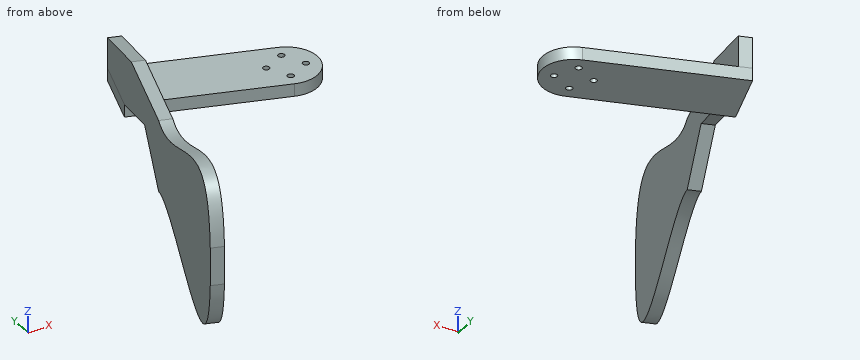
from build123d import *

# Parameters (mm, degrees)
SKETCH2_R           = 10
SKETCH2_R_2         = 1.275
BOSS_EXTRUDE1_DEPTH = 3
SKETCH3_R           = 1.275
BOSS_EXTRUDE2_DEPTH = 5
BOSS_EXTRUDE3_DEPTH = 5


with BuildPart() as part:
    # Sketch2 → Boss-Extrude1 (new body)
    with BuildSketch(Plane.XY):
        Circle(SKETCH2_R)
        with Locations((6.633008125, -2.236784122)):
            Circle(SKETCH2_R_2, mode=Mode.SUBTRACT)
        with Locations((-2.236784122, -6.633008125)):
            Circle(SKETCH2_R_2, mode=Mode.SUBTRACT)
        with Locations((-6.633008125, 2.236784122)):
            Circle(SKETCH2_R_2, mode=Mode.SUBTRACT)
        with Locations((2.236784122, 6.633008125)):
            Circle(SKETCH2_R_2, mode=Mode.SUBTRACT)
    extrude(amount=BOSS_EXTRUDE1_DEPTH)

    # Sketch3 → Boss-Extrude2 (add)
    with BuildSketch(Plane.XY.offset(3)):
        with BuildLine():
            Line((-3.994257361, -11.844657367), (-60.848612721, 7.327777966))
            Line((-60.848612721, 7.327777966), (-52.860097999, 31.0170927))
            Line((-52.860097999, 31.0170927), (3.994257361, 11.844657367))
            ThreePointArc((3.994257361, 11.844657367), (11.844657367, -3.994257361), (-3.994257361, -11.844657367))
        make_face()
        with Locations((6.633008125, -2.236784122)):
            Circle(SKETCH3_R, mode=Mode.SUBTRACT)
        with Locations((-2.236784122, -6.633008125)):
            Circle(SKETCH3_R, mode=Mode.SUBTRACT)
        with Locations((-6.633008125, 2.236784122)):
            Circle(SKETCH3_R, mode=Mode.SUBTRACT)
        with Locations((2.236784122, 6.633008125)):
            Circle(SKETCH3_R, mode=Mode.SUBTRACT)
    extrude(amount=-BOSS_EXTRUDE2_DEPTH)

    # Sketch4 → Boss-Extrude3 (add)
    with BuildSketch(Plane(origin=(-56.85435536, 19.172435333, 0), x_dir=(0.319540589, 0.947572589, 0), z_dir=(-0.947572589, 0.319540589, 0))):
        with BuildLine():
            Line((-62.942627893, -25.970573692), (-22.627671819, -25.970573692))
            Line((-22.627671819, -25.970573692), (12.5, -15.199288929))
            Line((12.5, -15.199288929), (12.5, -3))
            Line((12.5, -3), (-12.5, -3))
            Line((-12.5, -3), (-42.396291449, -12.167173681))
            Line((-42.396291449, -12.167173681), (-62.942627893, 2.349426308))
            add(Edge.make_bspline(
                [(-62.942627893, 2.349426308), (-87.492278411, -4.509248518), (-135.602543773, 45.42627104), (-139.208088658, -4.310573692)],
                knots=[0, 0, 0, 0, 1, 1, 1, 1], degree=3))
            Line((-139.208088658, -4.310573692), (-139.208088658, -19.310573692))
            add(Edge.make_bspline(
                [(-62.942627893, -25.970573692), (-87.492278411, -19.111898866), (-135.602543773, -69.047418424), (-139.208088658, -19.310573692)],
                knots=[0, 0, 0, 0, 1, 1, 1, 1], degree=3))
        make_face()
    extrude(amount=-BOSS_EXTRUDE3_DEPTH)


solid = part.part
The listing builds one solid part. Answer for the finished solid, in the listing's coordinates (mm). Give positions to 0.01 mm unless a question says otherwise; leave off trailing zeros. Write each loop counter-clockwise with the first axis right and the second up, starting at its lowest first coordinate (ties: lowest second). Pieces come first, ordered by that corner, then holes. Notation, with made-up numbers: (33, 68) - (79, 68) arc R26 cw to (79, 99) - close; hole circle Ø8 at (75.5, 0.25). An arc over 180 degrees is marked (long way). Use a Markdown table: item, result.
1. Section B-B on y = 15 is taken. Write down the section's boundary in (x, z).
Values follow:
| item | result |
|---|---|
| outline | (-58.26, -2) - (-5.36, -2) - (-5.36, 3) - (-52.98, 3) - (-52.98, 19.87) - (-58.26, 20.38) - close |
2. Find the intervals of material crossed by probe 1 along Z at (x, y) = (-9, -2.5); probe 2 along Z at (x, y) = (-53, 19); probe 3 along X at (y, z) = (-49, 18), in increasing order. Write a range as from..to.
Values follow:
| item | result |
|---|---|
| probe 1 | z = -2..3 |
| probe 2 | z = -2..18.7 |
| probe 3 | x = -79.84..-74.57 |
3. Section A-A on z = 1 is taken. Count the separate pieces of the cut face and the enclosed holes in it, plus the area to 3 significant figures.
Values follow:
| item | result |
|---|---|
| separate pieces | 2 |
| enclosed holes | 4 |
| area | 2,130 mm² |
4. Section C-C on x = -37.5 is taken. Write down the section's boundary in (y, z).
Values follow:
| item | result |
|---|---|
| outline | (-0.55, -2) - (25.84, -2) - (25.84, 3) - (-0.55, 3) - close |
5. Section D-D on y = -30 is taken. Write down the section's boundary in (x, z).
Values follow:
| item | result |
|---|---|
| outline | (-73.44, 5.46) - (-68.16, 6.65) - (-68.16, 25.97) - (-73.44, 25.97) - close |
6. Each of these flat-tipped pins is pushed along its axis until it touches: P1, Ø3, axis at y = -87.5, z = -5, coming from the -X side; P2, Ø6, axis at y = -65.5, z = 30, coming from the -X side; P3, Ø21, axis at x = -9.5, y = -1.5, coming from the +Z side. Where does it stop, or does it pass through?
Values follow:
| item | result |
|---|---|
| P1 | stops at x = -93.33 |
| P2 | stops at x = -86.42 |
| P3 | stops at z = 3 |
